Part model, mm, in its own coordinate system. A direction names the side the tool comes from. Round coordinates to 2 decimals unless told otherwise and drop trailing zeros. Return JSON: item names as keys, results as strings. Group by question number.
(1) Saw through at A-A (y = 0). State how many separate pieces and enclosed holes the cut face has, plus the area to 3 significant figures.
(2) Drop flat-ended pins along their axis: pin 1 Ø2 at (x, z) = (-10.5, -2) entering from -Y; pin 2 Ø3 at (x, y) = (-1.5, 4) entering from +Z; pin 3 Ø5.5 at (x, y) = (0, -0.5) entering from -Z; pin 4 Ø3.5 at (x, y) = (-6.74, -11.68) entering from +Z. Give the stop position or say it passes through.
(3) Tool access for faces 1 (the flat face through (2, 0, -2.642)), 2 (the flat face through (0, -2, 2.642)), 3 (the cylindrical face through (2.15, 5.58, 0.04)): list every direction of +Z, -Z, +X, -X, +Y, -Y with a clear straight run to the whole face (end or side of a thin tool).
(4) Mould opens along Y. For faces 4 (the cylindrical face through (16.111, 5.074, 1.969)), 5 (the cylindrical face through (10.236, 3.223, -3.206)), 6 (the flat face through (-11, -3, 3.81)) say: +Y half, -Y half, draft (parallel to the pull), parting line (faces both ways), or undercut.
(5) Drill centre lines: L1, parallel to X at y = -0.5, z = -2; L2, parallel to X at y = 1, z = -0.75; L3, parallel to Y at x = 0.5, z = 0.75. Where is each one in solid material? Low to high. Write a range as from..to.
from build123d import *

# Parameters (mm, degrees)
M4_CLEARANCE_HOLE1_D      = 4.3688
M4_CLEARANCE_HOLE2_D      = 4.3688
CHAMFER1_SIZE             = 0.254
CHAMFER2_SIZE             = 0.508
TAP_DRILL_FOR_4_40_TAP1_D = 2.2606
CUT_EXTRUDE1_DEPTH        = 25.743381025
CIRPATTERN1_COUNT         = 3


with BuildPart() as part:
    # Sketch1 → Revolve1 (revolve)
    with BuildSketch(Plane(origin=(0, 0, 0), x_dir=(1, 0, 0), z_dir=(0, 1, 0))):
        with BuildLine():
            Line((9.086103121, 2.6416), (0, 2.6416))
            Line((0, 2.6416), (0, -2.6416))
            Line((0, -2.6416), (9.086103121, -2.6416))
            Line((9.086103121, -2.6416), (9.271, -3.1496))
            Line((9.271, -3.1496), (10.7315, -2.618021473))
            Line((10.7315, -2.618021473), (10.7315, -3.81))
            Line((10.7315, -3.81), (16.891, -3.81))
            Line((16.891, -3.81), (16.891, -0.672020833))
            ThreePointArc((16.891, -0.672020833), (16.637, 0), (16.891, 0.672020833))
            Line((16.891, 0.672020833), (16.891, 3.81))
            Line((16.891, 3.81), (10.7315, 3.81))
            Line((10.7315, 3.81), (10.7315, 2.618021473))
            Line((10.7315, 2.618021473), (9.271, 3.1496))
            Line((9.271, 3.1496), (9.086103121, 2.6416))
        make_face()
    revolve(axis=Axis((0, 0, -3.81), (0, 0, 1)))

    # M4 Clearance Hole1 (through all)
    with Locations(Plane(origin=(0, 0, -3.81), x_dir=(-1, 0, 0), z_dir=(0, 0, -1))):
        with Locations((6.7437, -11.680431031), (6.7437, 11.680431031), (-6.7437, 11.680431031), (-13.4874, 0)):
            Hole(M4_CLEARANCE_HOLE1_D / 2)

    # M4 Clearance Hole2 (through all)
    with Locations(Plane.XY.offset(3.81)):
        with Locations((6.7437, -11.680431031), (-13.4874, 0)):
            Hole(M4_CLEARANCE_HOLE2_D / 2)

    # Chamfer1
    chamfer1_edges = [part.edges().sort_by_distance(p)[0] for p in [
        (11.303, 0, -3.81),
        (11.303, 0, 3.81),
        (4.5593, 11.680431031, -3.81),
        (4.5593, 11.680431031, 3.81),
        (-8.9281, 11.680431031, -3.81),
        (-8.9281, 11.680431031, 3.81),
        (-8.9281, -11.680431031, -3.81),
        (-8.9281, -11.680431031, 3.81),
        (-11.303, 0, 3.81),
        (-11.303, 0, -3.81),
        (8.9281, -11.680431031, 3.81),
        (8.9281, -11.680431031, -3.81),
    ]]
    chamfer(chamfer1_edges, length=CHAMFER1_SIZE)

    # Chamfer2
    chamfer2_edges = [part.edges().sort_by_distance(p)[0] for p in [
        (-16.891, 0, 3.81),
        (-16.891, 0, -3.81),
    ]]
    chamfer(chamfer2_edges, length=CHAMFER2_SIZE)

    # Tap Drill for #4-40 Tap1 (through all)
    with Locations(Plane(origin=(0, 0, -2.6416), x_dir=(-1, 0, 0), z_dir=(0, 0, -1))):
        with Locations((0, 0)):
            Hole(TAP_DRILL_FOR_4_40_TAP1_D / 2)

    # Sketch10 → Cut-Extrude1 (cut, through all)
    with BuildSketch(Plane.XY.offset(2.6416)):
        with BuildLine():
            ThreePointArc((6.426642817, -4.094223016), (7.62, 0), (6.426642817, 4.094223016))
            ThreePointArc((6.426642817, 4.094223016), (3.796426359, 4.677327966), (3.213321409, 2.047111508))
            ThreePointArc((3.213321409, 2.047111508), (3.81, 0), (3.213321409, -2.047111508))
            ThreePointArc((3.213321409, -2.047111508), (3.796426359, -4.677327966), (6.426642817, -4.094223016))
        make_face()
    cut_extrude1 = extrude(amount=-CUT_EXTRUDE1_DEPTH, mode=Mode.SUBTRACT)

    # CirPattern1: Cut-Extrude1 ×3 about axis
    cirpattern1_axis = Axis((0, 0, 0), (0, 0, 1))
    for i in range(1, CIRPATTERN1_COUNT):
        add(cut_extrude1.rotate(cirpattern1_axis, i * 360 / CIRPATTERN1_COUNT), mode=Mode.SUBTRACT)


solid = part.part
Computed values:
{
 "1": {"separate pieces": "5", "enclosed holes": "0", "area": "109 mm2"},
 "2": {"pin 1": "y = -13.97", "pin 2": "z = 2.64", "pin 3": "z = -2.64", "pin 4": "through"},
 "3": {"face 1": "-Z", "face 2": "+Z", "face 3": "+Z, -Z"},
 "4": {"face 4": "parting line", "face 5": "undercut", "face 6": "draft"},
 "5": {"L1": "-16.88..-15.61, -11.36..-1.01, 1.01..3.78, 7.6..11.36, 15.61..16.88", "L2": "-16.86..-15.43, -11.55..-6.04, -4.1..-0.53, 0.53..3.68, 7.55..11.55, 15.43..16.86", "L3": "-16.88..-7.6, -3.82..-1.01, 1.01..3.82, 7.6..16.88"}
}
